Job drawing, mm, ordinate dimensions from the low corner. One solid piece. A direction names the side the tool comes from. Round coordinates to 2 decimals unless told otherwise and drop trailing zeros. Write each loop counter-clockwise with the first axis right and the second up, starting at its lowest first coordinate (ties: lowest second). Pieces come first, ordered by that corner, then holes.
1) Saw through at C-C (x = 8.5). Write the cut outline in (y, z).
2) Which spindle directions (+Z, -Z, +X, -X, +Y, -Y) get a long thin tool onto all of the face, cutting with end or side? Do the marked faces 5, 6, 7, 8 and 9. Say none if no direction does.
3) Flat gauge pins, fed straight in: pin 1 (2 mm diameter, centred on x = 15, y = 3, fed in from +Z); pin 2 (10 mm diameter, centred on y = 6.5, z = 12, fed in from +X); pin 3 (1.6 mm diameter, centred on y = 1.5, z = 17.5, fed in from -X); pin 4 (5 mm diameter, centred on x = 8.5, z = 14.5, fed in from +Y). Where does each tip first touch, or does it go through?
4) Saw through at D-D (z = 2.5). Write the cut outline in (x, y), plus the area to 3 significant figures.
5) Pull direction Y, two halves, no side cores. Call the marked faces 1, 2, 3 and 4: +Y half, -Y half, draft (parallel to the pull), parting line (faces both ways), or undercut.
6) Saw through at B-B (y = 19.75). Write the cut outline in (x, z), plus the area to 3 significant figures.
7) Wall check: probe 1 along Y at (x, z) = (19, 10.75); probe 2 along X at (y, z) = (5.5, 9); probe 3 along X at (y, z) = (19.75, 4.75). Give the ranges that are in metal, low to high.
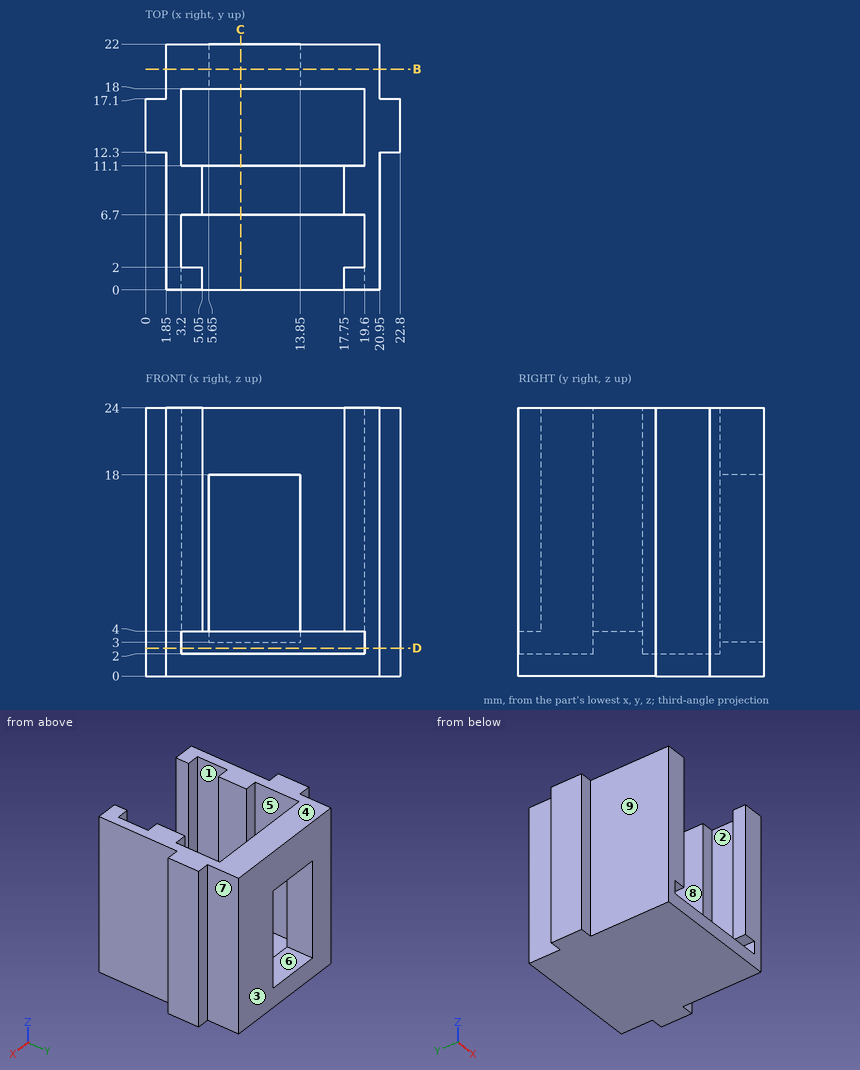
Evaluation:
1. outline: (0, 0) - (22, 0) - (22, 3) - (18, 3) - (18, 2) - (11.1, 2) - (11.1, 4) - (6.7, 4) - (6.7, 2) - (0, 2) - close; (18, 18) - (22, 18) - (22, 24) - (18, 24) - close
2. face 5: +Z
2. face 6: +Y
2. face 7: +Z, -Z, +X, +Y
2. face 8: +Z, -Y
2. face 9: +Z, -Z, -X, -Y
3. pin 1: stops at z = 2
3. pin 2: stops at x = 20.95
3. pin 3: stops at x = 1.85
3. pin 4: passes through
4. outline: (0, 12.3) - (1.85, 12.3) - (1.85, 0) - (3.2, 0) - (3.2, 6.7) - (19.6, 6.7) - (19.6, 0) - (20.95, 0) - (20.95, 12.3) - (22.8, 12.3) - (22.8, 17.1) - (20.95, 17.1) - (20.95, 22) - (1.85, 22) - (1.85, 17.1) - (0, 17.1) - close; hole (3.2, 11.1) - (19.6, 11.1) - (19.6, 18) - (3.2, 18) - close
4. area: 215 mm2
5. face 1: undercut
5. face 2: undercut
5. face 3: +Y half
5. face 4: draft
6. outline: (1.85, 0) - (20.95, 0) - (20.95, 24) - (1.85, 24) - close; hole (5.65, 3) - (13.85, 3) - (13.85, 18) - (5.65, 18) - close
6. area: 335 mm2
7. probe 1: y = 0 to 2, 6.7 to 11.1, 18 to 22
7. probe 2: x = 1.85 to 3.2, 19.6 to 20.95
7. probe 3: x = 1.85 to 5.65, 13.85 to 20.95
